Design review of the part built by this model. Coordinates are the model's own, in mm. A direction names the side the tool comes from. Give positions to 0.01 mm unless a question says otherwise; leave off trailing zeros. Write each loop counter-clockwise with the first axis right and the second up, starting at its lowest first coordinate (ties: lowest second). Pieces come first, ordered by that corner, then holes. Notation, with made-up numbers: (1.25, 89.25) -> (25.25, 89.25) arc R19 cw to (25.25, 98.25) -> close; hole circle Ø7 at (75.25, -8.5). An arc over 180 degrees is marked (long way). Return JSON: item names as keys, results as strings. Group by question number.
from build123d import *

# Parameters (mm, degrees)
SKETCH_1_W          = 52
SKETCH_1_H          = 46
SKETCH_1_R          = 1.75
EXTRUDE_2_DEPTH     = 4
SKETCH_2_W          = 46
SKETCH_2_H          = 42
SKETCH_2_R          = 2
SKETCH_2_R_2        = 13
EXTRUDE_3_DEPTH     = 4
SKETCH_4_R          = 12.5
CUT_EXTRUDE_1_DEPTH = 2
EXTRUDE_4_DEPTH     = 3
EXTRUDE_5_DEPTH     = 3
FILLET_1_R          = 3
FILLET_2_R          = 3
FILLET_3_R          = 3
FILLET_4_R          = 3
FILLET_5_R          = 3
FILLET_6_R          = 3
FILLET_7_R          = 3
FILLET_8_R          = 3
FILLET_9_R          = 1
FILLET_10_R         = 2


with BuildPart() as part:
    # 草图1 → 凸台-拉伸2 (new body)
    with BuildSketch(Plane(origin=(0, 0, 0), x_dir=(1, 0, 0), z_dir=(0, 1, 0))):
        Rectangle(SKETCH_1_W, SKETCH_1_H)
        with Locations((8, 0)):
            Circle(SKETCH_1_R, mode=Mode.SUBTRACT)
        with Locations((0, 8)):
            Circle(SKETCH_1_R, mode=Mode.SUBTRACT)
        with Locations((-8, 0)):
            Circle(SKETCH_1_R, mode=Mode.SUBTRACT)
        with Locations((0, -8)):
            Circle(SKETCH_1_R, mode=Mode.SUBTRACT)
    extrude(amount=EXTRUDE_2_DEPTH)

    # 草图2 → 凸台-拉伸3 (add)
    with BuildSketch(Plane.ZY.offset(26)):
        with Locations((0, 25)):
            Rectangle(SKETCH_2_W, SKETCH_2_H)
        with Locations((15.5, 40.5)):
            Circle(SKETCH_2_R, mode=Mode.SUBTRACT)
        with Locations((15.5, 9.5)):
            Circle(SKETCH_2_R, mode=Mode.SUBTRACT)
        with Locations((-15.5, 9.5)):
            Circle(SKETCH_2_R, mode=Mode.SUBTRACT)
        with Locations((-15.5, 40.5)):
            Circle(SKETCH_2_R, mode=Mode.SUBTRACT)
        with Locations((0, 25)):
            Circle(SKETCH_2_R_2, mode=Mode.SUBTRACT)
    extrude(amount=-EXTRUDE_3_DEPTH)

    # 草图4 → 切除-拉伸1 (cut)
    with BuildSketch(Plane(origin=(0, 4, 0), x_dir=(1, 0, 0), z_dir=(0, 1, 0))):
        Circle(SKETCH_4_R)
    extrude(amount=-CUT_EXTRUDE_1_DEPTH, mode=Mode.SUBTRACT)

    # 草图6 → 凸台-拉伸4 (add)
    with BuildSketch(Plane.XY.offset(23)):
        Polygon((-26, 46), (-22, 46), (-22, 24), (-2, 4), (26, 4), (26, 0), (-26, 0), align=None)
    extrude(amount=EXTRUDE_4_DEPTH)

    # 草图7 → 凸台-拉伸5 (add)
    with BuildSketch(Plane(origin=(0, 0, -23), x_dir=(-1, 0, 0), z_dir=(0, 0, -1))):
        Polygon((26, 46), (26, 0), (-26, 0), (-26, 4), (2, 4), (22, 24), (22, 46), align=None)
    extrude(amount=EXTRUDE_5_DEPTH)

    # 圆角1
    fillet_1_edges = [part.edges().sort_by_distance(p)[0] for p in [
        (-24, 46, 26),
    ]]
    fillet(fillet_1_edges, radius=FILLET_1_R)

    # 圆角2
    fillet_2_edges = [part.edges().sort_by_distance(p)[0] for p in [
        (-24, 46, -26),
    ]]
    fillet(fillet_2_edges, radius=FILLET_2_R)

    # 圆角3
    fillet_3_edges = [part.edges().sort_by_distance(p)[0] for p in [
        (26, 2, 26),
    ]]
    fillet(fillet_3_edges, radius=FILLET_3_R)

    # 圆角4
    fillet_4_edges = [part.edges().sort_by_distance(p)[0] for p in [
        (26, 2, -26),
    ]]
    fillet(fillet_4_edges, radius=FILLET_4_R)

    # 圆角5
    fillet_5_edges = [part.edges().sort_by_distance(p)[0] for p in [
        (-22, 24, 24.5),
    ]]
    fillet(fillet_5_edges, radius=FILLET_5_R)

    # 圆角6
    fillet_6_edges = [part.edges().sort_by_distance(p)[0] for p in [
        (-2, 4, 24.5),
    ]]
    fillet(fillet_6_edges, radius=FILLET_6_R)

    # 圆角7
    fillet_7_edges = [part.edges().sort_by_distance(p)[0] for p in [
        (-22, 24, -24.5),
    ]]
    fillet(fillet_7_edges, radius=FILLET_7_R)

    # 圆角8
    fillet_8_edges = [part.edges().sort_by_distance(p)[0] for p in [
        (-2, 4, -24.5),
    ]]
    fillet(fillet_8_edges, radius=FILLET_8_R)

    # 圆角9
    fillet_9_edges = [part.edges().sort_by_distance(p)[0] for p in [
        (-12.5, 4, 0),
    ]]
    fillet(fillet_9_edges, radius=FILLET_9_R)

    # 圆角10
    fillet_10_edges = [part.edges().sort_by_distance(p)[0] for p in [
        (-26, 0, 0),
    ]]
    fillet(fillet_10_edges, radius=FILLET_10_R)


solid = part.part
Q1. For L1, parallel to Y at x = -23.4, z = 15.5; L2, parallel to Z at x = 0, y = 1.1; L3, parallel to Y at x = -23, z = 0, list the stretches that pass through material, from the lowest coordinate up. Write a range as from..to.
Q2. Insertion check: pin 1 (2.5 mm diameter, centred on y = 9.5, z = 15.5, fed in from -X); pin 2 (4.5 mm diameter, centred on y = 9.5, z = -15.5, fed in from +X); pin 3 (12 mm diameter, centred on x = 5, z = -11, fed in from -Y); pin 4 (5 mm diameter, centred on x = 19.5, z = 16, fed in from +Y). Each pin has a flat end and moves straight along its axis. Give the tip position at first contact, or say it passes through.
Q3. Take a section at D-D, the plane z = -7. Count the separate pieces of the cut face and the enclosed holes in it, plus the area to 3 significant figures.
Q4. Take a section at A-A, the plane z = 15.5. Give the boundary of the cut face in (x, y), plus the area to 3 significant figures.
Q5. Take a section at B-B, the plane y = 36.5. Give the boundary of the cut face in (x, z), plus the area to 3 significant figures.
Q6. Tool access review of faces 4 (the face through (11.923, 2.507, -3.755)), 5 (the face through (-16, 10, 23)), 6 (the face through (-1.89, 4.22, -24.52)): name each direction out of +Z, -Z, +X, -X, +Y, -Y from which nothing blocks a thin tool from reaching the whole face with its end or side.
Q7. Mouldability with a two-part tool opening along X and no side actions: class faces 1 (the face through (-22, 34, -11)), 2 (the face through (-23.97, 45.14, 25.1)), 3 (the face through (1.617, 0.986, 8.67)) as +X half, -X half, draft (parallel to the pull), parting line (faces both ways), or undercut.
Q8. Take a section at C-C, the plane y = 29. Give the boundary of the cut face in (x, z), plus the area to 3 significant figures.
Final values:
{
 "1": {"L1": "y = 0..7.5, 11.5..38.5, 42.5..46", "L2": "z = -26..-9.75, -6.25..6.25, 9.75..26", "L3": "y = 0..12, 38..46"},
 "2": {"pin 1": "passes through", "pin 2": "stops at x = -22", "pin 3": "stops at y = 0", "pin 4": "stops at y = 4"},
 "3": {"separate pieces": "3", "enclosed holes": "0", "area": "240 mm²"},
 "4": {"outline": "(-26, 2) arc R2 ccw to (-24, 0) -> (26, 0) -> (26, 4) -> (-22, 4) -> (-22, 7.5) -> (-26, 7.5) -> close; (-26, 11.5) -> (-22, 11.5) -> (-22, 38.5) -> (-26, 38.5) -> close; (-26, 42.5) -> (-22, 42.5) -> (-22, 46) -> (-26, 46) -> close", "area": "343 mm²"},
 "5": {"outline": "(-26, -26) -> (-22, -26) -> (-22, -6.06) -> (-26, -6.06) -> close; (-26, 6.06) -> (-22, 6.06) -> (-22, 26) -> (-26, 26) -> close", "area": "160 mm²"},
 "6": {"face 4": "+Y", "face 5": "+X, +Y", "face 6": "+Z, -Z, +X, +Y"},
 "7": {"face 1": "+X half", "face 2": "draft", "face 3": "undercut"},
 "8": {"outline": "(-26, -26) -> (-22, -26) -> (-22, -12.37) -> (-26, -12.37) -> close; (-26, 12.37) -> (-22, 12.37) -> (-22, 26) -> (-26, 26) -> close", "area": "109 mm²"}
}
